Here's how the part is built. I have some questions about the finished solid (model axes, mm). Round coordinates to 2 decimals unless told otherwise and drop trailing zeros. Write each loop counter-clockwise with the first axis right and the second up, starting at its lowest first coordinate (ties: lowest second). Pieces come first, ordered by that corner, then holes. Notation, with made-up numbers: (36, -1.75) -> (71, -1.75) arc R24 cw to (71, 24.25) -> close; hole circle Ø11 at (48.5, 74). An arc over 180 degrees is marked (long way). Put each result on its own line as item: value. Start each with the question number.
1) Will these pins go through, and if not, where does the flat tip stop? P1, Ø18, axis at x = 0, z = 0, coming from the +Y side; P2, Ø3, axis at y = 2.5, z = -100, coming from the -X side; P3, Ø1.5, axis at x = 19, y = 4, coming from the -Z side.
2) I want a section at B-B, the plane z = 0. List the corners of the cut face in (x, y) for me, then the cut area to 4 significant figures.
3) If I drill on line 1 along X through (y, z) = (1.05, 0); line 2 along Z through (x, y) = (-4, 3.15); line 3 along Z through (x, y) = (-91, 0.45), over which ranges is the centre line in solid material (lowest first)? Write a range as [from, to].
4) I want a section at D-D, the plane x = -105.5. List the corners of the cut face in (y, z) for me, then the cut area to 3 significant figures.
5) We'd pull the mould along X, two halves only. Please class faces 1 (the cylindrical face through (0.66, 2.465, -14.985)), 2 (the flat face through (-31, 0, -2)), 3 (the cylindrical face through (-143.99, 2.46, -31.98)): released by +X, released by -X, zero draft, split by the parting line, or undercut.
6) I want a section at C-C, the plane y = 2.85. Give the number of separate pieces and of enclosed holes in the cut face, then the cut area to 3 significant figures.
7) I want a section at A-A, the plane x = 0. List the corners of the cut face in (y, z) for me.
from build123d import *

# Parameters (mm, degrees)
ESQUISSE1_R        = 147.5
ESQUISSE1_R_2      = 15
ESQUISSE1_R_3      = 3
ESQUISSE1_R_4      = 1.5
BOSS_EXTRU_1_DEPTH = 5


with BuildPart() as part:
    # Esquisse1 → Boss.-Extru.1 (new body)
    with BuildSketch(Plane(origin=(0, 0, 0), x_dir=(1, 0, 0), z_dir=(0, 1, 0))):
        with Locations(Location((0, 0, 0), (0, 0, 270))):
            Circle(ESQUISSE1_R)
        with Locations(Location((0, 0, 0), (0, 0, 270))):
            Circle(ESQUISSE1_R_2, mode=Mode.SUBTRACT)
        with Locations(Location((-13.540108487, 90.127070907, 0), (0, 0, 270))):
            Circle(ESQUISSE1_R_3, mode=Mode.SUBTRACT)
        with Locations(Location((-82.082198921, 39.607272923, 0), (0, 0, 270))):
            Circle(ESQUISSE1_R_3, mode=Mode.SUBTRACT)
        with Locations(Location((75.342010962, 51.281622754, 0), (0, 0, 270))):
            Circle(ESQUISSE1_R_3, mode=Mode.SUBTRACT)
        with Locations(Location((84.822389485, -33.337451765, 0), (0, 0, 270))):
            Circle(ESQUISSE1_R_3, mode=Mode.SUBTRACT)
        with Locations(Location((6.740188753, -90.888906384, 0), (0, 0, 270))):
            Circle(ESQUISSE1_R_3, mode=Mode.SUBTRACT)
        with Locations(Location((-71.282271006, -56.78962307, 0), (0, 0, 270))):
            Circle(ESQUISSE1_R_3, mode=Mode.SUBTRACT)
        with Locations(Location((-20.889727943, -47.797718878, 0), (0, 0, 270))):
            Circle(ESQUISSE1_R_4, mode=Mode.SUBTRACT)
        with Locations(Location((-30.949170814, 41.989892072, 0), (0, 0, 270))):
            Circle(ESQUISSE1_R_4, mode=Mode.SUBTRACT)
    extrude(amount=BOSS_EXTRU_1_DEPTH)


solid = part.part
Findings:
1. P1: passes through
1. P2: stops at x = -109.79
1. P3: stops at z = -146.37
2. outline: (-147.5, 0) -> (-15, 0) -> (-15, 5) -> (-147.5, 5) -> close; (15, 0) -> (147.5, 0) -> (147.5, 5) -> (15, 5) -> close
2. area: 1,325 mm2
3. line 1: x = [-147.5, -15], [15, 147.5]
3. line 2: z = [-147.45, -14.46], [14.46, 147.45]
3. line 3: z = [-116.08, 116.08]
4. outline: (0, -103.08) -> (5, -103.08) -> (5, 103.08) -> (0, 103.08) -> close
4. area: 1,030 mm2
5. face 1: undercut
5. face 2: zero draft
5. face 3: split by the parting line
6. separate pieces: 1
6. enclosed holes: 9
6. area: 67,500 mm2
7. outline: (0, -147.5) -> (5, -147.5) -> (5, -15) -> (0, -15) -> close; (0, 15) -> (5, 15) -> (5, 147.5) -> (0, 147.5) -> close
